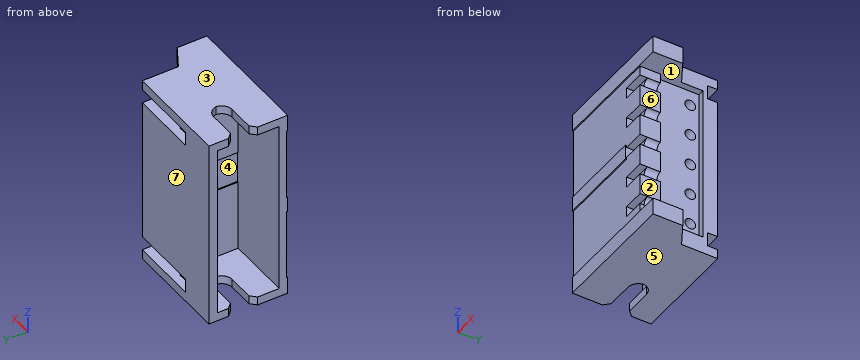
from build123d import *

# Parameters (mm, degrees)
SKETCH_1_W               = 6
SKETCH_1_H               = 3.7
EXTRUDE_1_DEPTH          = 9
SKETCH_2_W               = 1.993366308
SKETCH_2_H               = 0.87
CUT_EXTRUDE_1_DEPTH      = 12.431972708
CHAMFER_1_SIZE           = 0.25
FILLET_1_R               = 0.5
SKETCH_3_W               = 8.2
SKETCH_3_H               = 2.9
CUT_EXTRUDE_2_DEPTH      = 2.8
SKETCH_4_W               = 7.4
SKETCH_4_H               = 3
CUT_EXTRUDE_3_DEPTH      = 1.05
SKETCH_5_W               = 7.4
SKETCH_5_H               = 2
CUT_EXTRUDE_4_DEPTH      = 0.3
SKETCH_6_R               = 0.25
CUT_EXTRUDE_5_DEPTH      = 1
SKETCH_7_R               = 0.25
CUT_EXTRUDE_6_DEPTH      = 11.784827305
SKETCH_8_W               = 1
SKETCH_8_H               = 0.5
CUT_EXTRUDE_7_DEPTH      = 0.4
CUT_EXTRUDE_8_DEPTH      = 12.431972708
CUT_EXTRUDE_8_DEPTH_BACK = 0.05
SKETCH_10_W              = 0.66
SKETCH_10_H              = 0.49
CUT_EXTRUDE_9_DEPTH      = 3.2
SKETCH_11_W              = 8.2
SKETCH_11_H              = 1.5
CUT_EXTRUDE_10_DEPTH     = 0.25
SKETCH_12_W              = 1.5
SKETCH_12_H              = 1.5
CUT_EXTRUDE_11_DEPTH     = 0.05
CHAMFER_2_SIZE           = 0.3


# Some blends are built 0.0001 mm under size
with BuildPart() as part:
    # 스케치1 → 보스-돌출1 (new body)
    with BuildSketch(Plane.XY):
        with Locations((3, 1.85)):
            Rectangle(SKETCH_1_W, SKETCH_1_H)
    extrude(amount=EXTRUDE_1_DEPTH)

    # 스케치2 → 컷-돌출1 (cut, through all)
    with BuildSketch(Plane.XY.offset(9)):
        Polygon((6, 3.7), (4.95, 3.7), (4.95, 2), (6, 1.393782217), align=None)
        with Locations((0.996683154, 2.1)):
            Rectangle(SKETCH_2_W, SKETCH_2_H)
    extrude(amount=-CUT_EXTRUDE_1_DEPTH, mode=Mode.SUBTRACT)

    # 모따기1
    chamfer_1_edges = [part.edges().sort_by_distance(p)[0] for p in [
        (0, 1.665, 4.5),
        (0, 2.535, 4.5),
    ]]
    chamfer(chamfer_1_edges, length=CHAMFER_1_SIZE)

    # 필렛1
    # the kernel refuses this fillet: 0.5 mm, written as the material it adds along each edge
    with BuildSketch(Plane(origin=(1.993366308, 1.665, 9), x_dir=(-1, 0, 0), z_dir=(0, 0, -1)), Plane(origin=(1.993366308, 2.535, 9), x_dir=(0, -1, 0), z_dir=(0, 0, -1))) as fillet_1_piece_1:
        with BuildLine():
            CenterArc((FILLET_1_R, FILLET_1_R), FILLET_1_R, 180, 90)
            Line((0, FILLET_1_R), (0, 0))
            Line((0, 0), (FILLET_1_R, 0))
        make_face()
    extrude(amount=9)

    # 스케치3 → 컷-돌출2 (cut)
    with BuildSketch(Plane.ZY):
        with Locations((4.5, 1.85)):
            Rectangle(SKETCH_3_W, SKETCH_3_H)
    extrude(amount=-CUT_EXTRUDE_2_DEPTH, mode=Mode.SUBTRACT)

    # 스케치4 → 컷-돌출3 (cut)
    with BuildSketch(Plane(origin=(6, 0, 0), x_dir=(0, 0, -1), z_dir=(1, 0, 0))):
        with Locations((-4.5, 1.5)):
            Rectangle(SKETCH_4_W, SKETCH_4_H)
    extrude(amount=-CUT_EXTRUDE_3_DEPTH, mode=Mode.SUBTRACT)

    # 스케치5 → 컷-돌출4 (cut)
    with BuildSketch(Plane(origin=(4.95, 0, 0), x_dir=(0, 0, -1), z_dir=(1, 0, 0))):
        with Locations((-4.5, 2)):
            Rectangle(SKETCH_5_W, SKETCH_5_H)
    extrude(amount=-CUT_EXTRUDE_4_DEPTH, mode=Mode.SUBTRACT)

    # 스케치6 → 컷-돌출5 (cut)
    with BuildSketch(Plane.XZ):
        with Locations((4.95, 4.5)):
            Circle(SKETCH_6_R)
        with Locations((4.95, 6)):
            Circle(SKETCH_6_R)
        with Locations((4.95, 3)):
            Circle(SKETCH_6_R)
        with Locations((4.95, 7.5)):
            Circle(SKETCH_6_R)
        with Locations((4.95, 1.5)):
            Circle(SKETCH_6_R)
    extrude(amount=-CUT_EXTRUDE_5_DEPTH, mode=Mode.SUBTRACT)

    # 스케치7 → 컷-돌출6 (cut, through all)
    with BuildSketch(Plane(origin=(4.65, 0, 0), x_dir=(0, 0, -1), z_dir=(1, 0, 0))):
        with Locations((-7.5, 2.6)):
            Circle(SKETCH_7_R)
        with Locations((-6, 2.6)):
            Circle(SKETCH_7_R)
        with Locations((-4.5, 2.6)):
            Circle(SKETCH_7_R)
        with Locations((-3, 2.6)):
            Circle(SKETCH_7_R)
        with Locations((-1.5, 2.6)):
            Circle(SKETCH_7_R)
    extrude(amount=-CUT_EXTRUDE_6_DEPTH, mode=Mode.SUBTRACT)

    # 스케치8 → 컷-돌출7 (cut)
    with BuildSketch(Plane.XZ):
        with Locations((4.45, 7.5)):
            Rectangle(SKETCH_8_W, SKETCH_8_H)
        with Locations((4.45, 6)):
            Rectangle(SKETCH_8_W, SKETCH_8_H)
        with Locations((4.45, 4.5)):
            Rectangle(SKETCH_8_W, SKETCH_8_H)
        with Locations((4.45, 3)):
            Rectangle(SKETCH_8_W, SKETCH_8_H)
        with Locations((4.45, 1.5)):
            Rectangle(SKETCH_8_W, SKETCH_8_H)
    extrude(amount=-CUT_EXTRUDE_7_DEPTH, mode=Mode.SUBTRACT)

    # 스케치9 → 컷-돌출8 (cut, two sides: drawn at the far end of the back side and taken through both)
    with BuildSketch(Plane.XZ.offset(-CUT_EXTRUDE_8_DEPTH_BACK)):
        Polygon((4.95, 8.2), (0, 8.2), (0, 4.85), (3.95, 4.85), (3.95, 4.75), (4.95, 4.75), (4.95, 5.75), (3.95, 5.75), (3.95, 6.25), (4.95, 6.25), (4.95, 7.25), (3.95, 7.25), (3.95, 7.75), (4.95, 7.75), align=None)
        Polygon((3.95, 4.15), (0, 4.15), (0, 0.8), (4.95, 0.8), (4.95, 1.25), (3.95, 1.25), (3.95, 1.75), (4.95, 1.75), (4.95, 2.75), (3.95, 2.75), (3.95, 3.25), (4.95, 3.25), (4.95, 4.25), (3.95, 4.25), align=None)
    extrude(amount=CUT_EXTRUDE_8_DEPTH + CUT_EXTRUDE_8_DEPTH_BACK, mode=Mode.SUBTRACT)

    # 스케치10 → 컷-돌출9 (cut)
    with BuildSketch(Plane(origin=(4.95, 0, 0), x_dir=(0, 0, -1), z_dir=(1, 0, 0))):
        with Locations((-8.22, 3.455)):
            Rectangle(SKETCH_10_W, SKETCH_10_H)
        with Locations((-0.78, 3.455)):
            Rectangle(SKETCH_10_W, SKETCH_10_H)
    extrude(amount=-CUT_EXTRUDE_9_DEPTH, mode=Mode.SUBTRACT)

    # 스케치11 → 컷-돌출10 (cut)
    with BuildSketch(Plane.ZY.offset(-2.8)):
        with Locations((4.5, 1.15)):
            Rectangle(SKETCH_11_W, SKETCH_11_H)
    extrude(amount=-CUT_EXTRUDE_10_DEPTH, mode=Mode.SUBTRACT)

    # 스케치12 → 컷-돌출11 (cut)
    with BuildSketch(Plane.ZY.offset(-3.05)):
        with Locations((4.5, 1.15)):
            Rectangle(SKETCH_12_W, SKETCH_12_H)
    extrude(amount=-CUT_EXTRUDE_11_DEPTH, mode=Mode.SUBTRACT)

    # 모따기2
    chamfer_2_edges = [part.edges().sort_by_distance(p)[0] for p in [
        (2.8, 1.9, 4.5),
    ]]
    chamfer(chamfer_2_edges, length=CHAMFER_2_SIZE - 0.0001)  # a hair under: the kernel refuses the full size


solid = part.part
The listing builds one solid part. Answer for the finished solid, in the listing's coordinates (mm). Face numbers are marked on the shaded views. A direction names the side the tool comes from. Give positions to 0.01 mm unless a question says otherwise; leave off trailing zeros. Loops run counter-clockwise (first coordinate to the right, second up) from the corner with the lowest first, then second, coordinate; pieces in that order, holes last.
Item 1: This flat-tipped pin is pushed along its axis until it touches: pin 1 Ø1 at (y, z) = (0.5, 6.5) entering from +X. Where does it stop, or does it pass through?
Derived:
pin 1: stops at x = 4.95
Item 2: A cutting plane is placed at C-C (z = 5.5). Give the vertices of the cut face in (x, y).
Derived:
outline: (0, 0.05) - (4.95, 0.05) - (4.95, 1) - (4.65, 1) - (4.65, 3) - (4.95, 3) - (4.95, 3.7) - (0, 3.7) - (0, 3.3) - (2.8, 3.3) - (2.8, 2.2) - (3.05, 1.95) - (3.05, 0.4) - (0, 0.4) - close
Item 3: A cutting plane is placed at D-D (y = 0.8). Give the vertices of the cut face in (x, z), then the cut area to 3 significant figures.
Derived:
outline: (0, 0) - (6, 0) - (6, 0.8) - (4.95, 0.8) - (4.95, 1.25) arc R0.25 cw to (4.95, 1.75) - (4.95, 2.75) arc R0.25 cw to (4.95, 3.25) - (4.95, 4.25) arc R0.25 cw to (4.95, 4.75) - (4.95, 5.75) arc R0.25 cw to (4.95, 6.25) - (4.95, 7.25) arc R0.25 cw to (4.95, 7.75) - (4.95, 8.2) - (6, 8.2) - (6, 9) - (0, 9) - (0, 8.6) - (3.05, 8.6) - (3.05, 5.25) - (3.1, 5.25) - (3.1, 3.75) - (3.05, 3.75) - (3.05, 0.4) - (0, 0.4) - close
area: 20.7 mm2
Item 4: Find the intervals of material crossed by line 1 along Y through (x, z) = (2.1, 6.5); line 2 along Y through (x, z) = (4.05, 7.5); line 3 along Z through (x, y) = (5, 0.65), in increasing order.
Derived:
line 1: y = 0.05 to 0.4, 3.3 to 3.7
line 2: y = 0.4 to 2.35, 2.85 to 3.7
line 3: z = 0 to 0.8, 8.2 to 9
Item 5: A cutting plane is placed at B-B (z = 1.5). Give the vertices of the cut face in (x, y), then the cut area to 3 significant figures.
Derived:
outline: (0, 0.05) - (3.95, 0.05) - (3.95, 0.4) - (4.7, 0.4) - (4.7, 1) - (4.65, 1) - (4.65, 2.35) - (2.8, 2.35) - (2.8, 2.2) - (3.05, 1.95) - (3.05, 0.4) - (0, 0.4) - close; (0, 3.3) - (2.8, 3.3) - (2.8, 2.85) - (4.65, 2.85) - (4.65, 3) - (4.95, 3) - (4.95, 3.7) - (0, 3.7) - close
area: 7.50 mm2
Item 6: Determine the mould class of the marked faces 5, 6 and 7 for opening direction Z: +Z half, -Z half, draft (parallel to the pull), parting line (faces both ways), or undercut.
Derived:
face 5: -Z half
face 6: undercut
face 7: draft
Item 7: A cutting plane is placed at A-A (x = 0.75). Give the vertices of the cut face in (y, z) (3 decimals), then the cut area to 3 significant figures.
Derived:
outline: (0, 0) - (1.665, 0) - (1.665, 0.4) - (0.4, 0.4) - (0.4, 8.6) - (1.665, 8.6) - (1.665, 9) - (0, 9) - (0, 8.2) - (0.05, 8.2) - (0.05, 4.85) - (0, 4.85) - (0, 4.15) - (0.05, 4.15) - (0.05, 0.8) - (0, 0.8) - close; (2.535, 0) - (3.7, 0) - (3.7, 9) - (2.535, 9) - (2.535, 8.6) - (3.3, 8.6) - (3.3, 0.4) - (2.535, 0.4) - close
area: 8.49 mm2
Item 8: A tool of negligible diameter and unlimited length cuts with its end or side. For the marked faces 1, 2, 3 and 4, from which of +Z, -Z, +X, -X, +Y, -Y can it reach the whole face along a straight path? Write none if from no direction.
Derived:
face 1: +X
face 2: +X, +Y, -Y
face 3: +Z, +X, -X, +Y, -Y
face 4: -X
